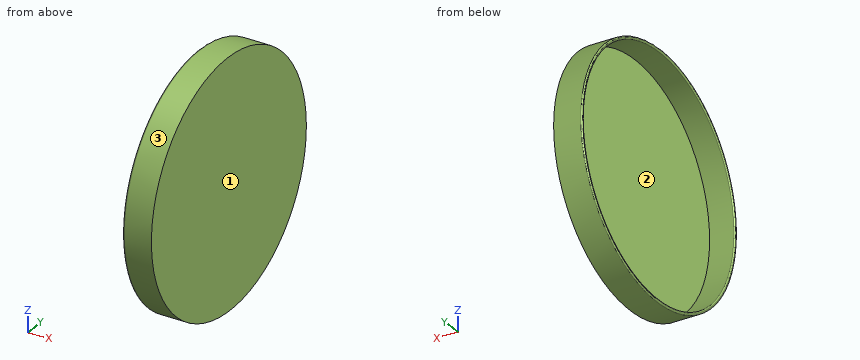
from build123d import *

# Parameters (mm, degrees)
F0_R     = 107.95
F1_DEPTH = 25
F2_T     = -2.5
F3_R     = 1


with BuildPart() as f1:
    # F0 (on Right) → F1 (new body)
    with BuildSketch(Plane.YZ):
        Circle(F0_R)
    extrude(amount=F1_DEPTH)

    # F2
    f2_openings = [f1.faces().sort_by_distance(p)[0] for p in [
        (0, 0, 0),
    ]]
    offset(amount=F2_T, openings=f2_openings)

    # F3
    f3_edges = [f1.edges().sort_by_distance(p)[0] for p in [
        (0, -107.95, 0),
        (0, -105.45, 0),
    ]]
    fillet(f3_edges, radius=F3_R)


solid = f1.part
Input: part model. Units: mm. Frame: model coordinates. Face numbers are marked on the shaded views. Coordinates: 2 decimals unless noted, no trailing zeros. Loops run counter-clockwise (first coordinate to the right, second up) from the corner with the lowest first, then second, coordinate; pieces in that order, holes last. Notation, with made-up numbers: (12.25, 70.5) -> (58.25, 70.5) arc R14 cw to (58.25, 95.5) -> close; hole circle Ø9 at (33, -4.75). An arc over 180 degrees is marked (long way). One line per item, written item: value.
(1) Pin query (flat end, axial travel): pin 1 Ø12 at (x, y) = (16, -69) entering from -Z; pin 2 Ø2 at (y, z) = (-16, -1.5) entering from -X; pin 3 Ø12 at (x, y) = (20, -37) entering from -Z. Return the tip coordinate at first contact, or that it passes through.
Answer below:
pin 1: stops at z = -87.66
pin 2: stops at x = 22.5
pin 3: stops at z = -103.4
(2) Cut plane A-A (z = 0). Output: boundary loops of the cut face in (x, y), then the cut area to 3 significant figures.
Answer below:
outline: (0, -106.95) arc R1 ccw to (1, -107.95) -> (25, -107.95) -> (25, 107.95) -> (1, 107.95) arc R1 ccw to (0, 106.95) -> (0, 106.45) arc R1 ccw to (1, 105.45) -> (22.5, 105.45) -> (22.5, -105.45) -> (1, -105.45) arc R1 ccw to (0, -106.45) -> close
area: 651 mm2
(3) Draft query along Y for the marked faces 1, 2 and 3. Return one class per face: pulls with the +Y half, pulls with the -Y half, needs draft (parallel to the pull), parting line crosses it, or undercut.
Answer below:
face 1: needs draft
face 2: undercut
face 3: parting line crosses it
(4) Ray query, line 1 along Z through (x, y) = (10.5, 0); line 2 along X through (y, z) = (61, 8); line 3 along Z through (x, y) = (5.75, 45.5). Return the intervals inside material, ascending.
Answer below:
line 1: z = -107.95 to -105.45, 105.45 to 107.95
line 2: x = 22.5 to 25
line 3: z = -97.89 to -95.13, 95.13 to 97.89
(5) Cut plane C-C (x = 9.5). Output: boundary loops of the cut face in (y, z), then the cut area to 3 significant figures.
Answer below:
outline: circle Ø215.9 at (0, 0); hole circle Ø210.9 at (0, 0)
area: 1,680 mm2
